For this review, take the finished solid that the model builds, in its own axes (mm). Coordinates: 2 decimals unless noted, no trailing zeros. Write each loop counter-clockwise with the first axis right and the second up, starting at its lowest first coordinate (ties: lowest second). Pieces come first, ordered by that corner, then holes.
```python
from build123d import *

# Parameters (mm, degrees)
SKETCH1_R              = 10
BOSS_EXTRUDE1_DEPTH    = 2.5
CUT_EXTRUDE1_OUTLINE_R = 1.5
CUT_EXTRUDE1_DEPTH     = 2.5


# Read off the part's stored shape, not the designer's step: Cut-Extrude1
with BuildPart() as part:
    # Sketch1 → Boss-Extrude1 (new body)
    with BuildSketch(Plane.XY):
        Circle(SKETCH1_R)
        Polygon((-2.644215925, 1.298692578), (-2.51581008, 0.894119117), (-2.870737377, 0.661322297), (-2.883640833, 0.599227456), (-2.896544289, 0.537132615), (-2.663747469, 0.182205319), (-2.942705268, -0.137717003), (-2.938377242, -0.20099051), (-2.934049215, -0.264264016), (-2.614126893, -0.543221815), (-2.796426171, -0.926542463), (-2.775187652, -0.986301929), (-2.753949133, -1.046061394), (-2.370628485, -1.228360672), (-2.442748938, -1.646650507), (-2.40617509, -1.698463845), (-2.369601242, -1.750277184), (-1.951311407, -1.822397637), (-1.907904191, -2.244634016), (-1.858707529, -2.284658469), (-1.809510867, -2.324682922), (-1.387274489, -2.281275706), (-1.231558919, -2.676143288), (-1.173388134, -2.701410425), (-1.115217349, -2.726677563), (-0.720349768, -2.570961993), (-0.463874555, -2.909175255), (-0.401043909, -2.917811129), (-0.338213262, -2.926447002), (0, -2.669971789), (0.338213262, -2.926447002), (0.401043909, -2.917811129), (0.463874555, -2.909175255), (0.720349768, -2.570961993), (1.115217349, -2.726677563), (1.173388134, -2.701410425), (1.231558919, -2.676143288), (1.387274489, -2.281275706), (1.809510867, -2.324682922), (1.858707529, -2.284658469), (1.907904191, -2.244634016), (1.951311407, -1.822397637), (2.369601242, -1.750277184), (2.40617509, -1.698463845), (2.442748938, -1.646650507), (2.370628485, -1.228360672), (2.753949133, -1.046061394), (2.775187652, -0.986301929), (2.796426171, -0.926542463), (2.614126893, -0.543221815), (2.934049215, -0.264264016), (2.938377242, -0.20099051), (2.942705268, -0.137717003), (2.663747469, 0.182205319), (2.896544289, 0.537132615), (2.883640833, 0.599227456), (2.870737377, 0.661322297), (2.51581008, 0.894119117), (2.644215925, 1.298692578), (2.615037976, 1.355003462), (2.585860027, 1.411314347), (2.181286567, 1.539720192), (2.195778161, 1.963934453), (2.152489715, 2.010285061), (2.109201269, 2.056635669), (1.684987008, 2.071127263), (1.584489576, 2.483520294), (1.530301139, 2.516473013), (1.476112702, 2.549425731), (1.063719671, 2.4489283), (0.855686648, 2.818914796), (0.794617128, 2.836025673), (0.733547608, 2.85313655), (0.363561112, 2.645103528), (0.063421356, 2.945243283), (0, 2.945243283), (-0.063421356, 2.945243283), (-0.363561112, 2.645103528), (-0.733547608, 2.85313655), (-0.794617128, 2.836025673), (-0.855686648, 2.818914796), (-1.063719671, 2.4489283), (-1.476112702, 2.549425731), (-1.530301139, 2.516473013), (-1.584489576, 2.483520294), (-1.684987008, 2.071127263), (-2.109201269, 2.056635669), (-2.152489715, 2.010285061), (-2.195778161, 1.963934453), (-2.181286567, 1.539720192), (-2.585860027, 1.411314347), (-2.615037976, 1.355003462), align=None, mode=Mode.SUBTRACT)
    extrude(amount=BOSS_EXTRUDE1_DEPTH)

    # Cut-Extrude1 outline → Cut-Extrude1 (cut)
    with BuildSketch(Plane.XY):
        with Locations((-6, 0)):
            Circle(CUT_EXTRUDE1_OUTLINE_R)
    extrude(amount=CUT_EXTRUDE1_DEPTH, mode=Mode.SUBTRACT)


solid = part.part
```
Q1. Add section A-A (x = -6). State the section outline as (y, z) points.
Ans:
outline: (-8, 0) - (-1.5, 0) - (-1.5, 2.5) - (-8, 2.5) - close; (1.5, 0) - (8, 0) - (8, 2.5) - (1.5, 2.5) - close
Q2. Add section D-D (x = 4.5). State the section outline as (y, z) points.
Ans:
outline: (-8.93, 0) - (8.93, 0) - (8.93, 2.5) - (-8.93, 2.5) - close
Q3. For probe 1 along Y at (x, z) = (-6, 1.55); probe 2 along Y at (x, z) = (2.25, 0.25); probe 3 along X at (y, z) = (-2.5, 0.25), list the stretches that pass through material, from the lowest coordinate up.
Ans:
probe 1: y = -8 to -1.5, 1.5 to 8
probe 2: y = -9.74 to -1.77, 1.52 to 9.74
probe 3: x = -9.68 to -1.3, 1.3 to 9.68
Q4. Draft analysis for pull direction Y (two halves, no side actions). For faces 1 (the flat face through (2.1, -2.1, 0)), 2 (the cylindrical face through (-2.17, -9.76, 1.23)), 3 (the cylindrical face through (-7.2, -0.9, 1.2)), state which applies: +Y half, -Y half, draft (parallel to the pull), parting line (faces both ways), or undercut.
Ans:
face 1: draft
face 2: parting line
face 3: undercut
Q5. Add section B-B (z = 1.4). Give the number of separate pieces and of enclosed holes in the cut face, then the cut area to 3 significant figures.
Ans:
separate pieces: 1
enclosed holes: 2
area: 282 mm2
Q6. Add section C-C (y = 8). State the section outline as (x, z) points.
Ans:
outline: (-6, 0) - (6, 0) - (6, 2.5) - (-6, 2.5) - close
Q7. Clearance check with flat-ended pins moving along their axes: pin 1 Ø1.5 at (y, z) = (2, 0.5) entering from +X; pin 2 Ø5 at (x, y) = (6.5, -1) entering from -Z. State where each tip first meets the part, or that it passes through.
Ans:
pin 1: stops at x = 9.92
pin 2: stops at z = 0
